Can you work these out from the model? Positions are in its coordinate system, mm. Face numbers are marked on the shaded views. A direction names the side the tool comes from. Round coordinates to 2 decimals unless told otherwise and drop trailing zeros. Order: outer loops, then holes, each group sorted by start corner. A loop starts at its lowest first (then second) coordinate and runs counter-clockwise, first axis right, second up. Notation, with made-up numbers: M -23.75,22 L 33.25,22 A25 cw 33.25,35 Z; hole C -2.5,6 d11. An arc over 180 degrees is marked long. One line per question, with ' | ' between items.
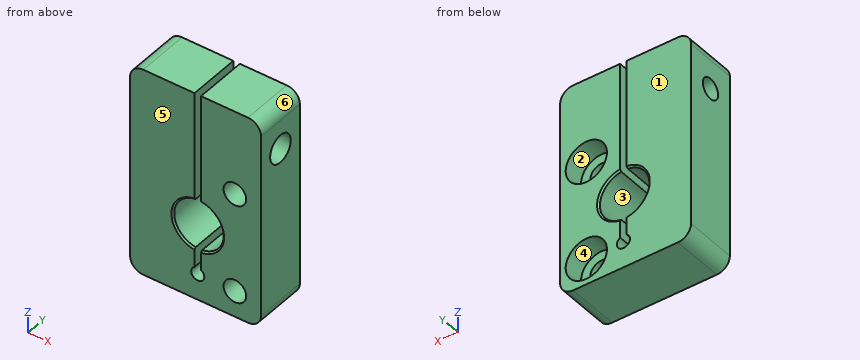
```python
from build123d import *

# Parameters (mm, degrees)
SKETCH1_W                            = 12.7
SKETCH1_H                            = 31.75
EXTRUDE1_DEPTH                       = 25.4
CBORE_FOR_M5_SHCS1_D                 = 5.5
CBORE_FOR_M5_SHCS1_DEPTH             = 12.7
CBORE_FOR_M5_SHCS1_CBORE_D           = 10
CBORE_FOR_M5_SHCS1_CBORE_DEPTH       = 5
CUT_EXTRUDE1_REACH                   = 14.7
F_17_64_0_26563_DIAMETER_HOLE1_D     = 6.747002
F_17_64_0_26563_DIAMETER_HOLE1_DEPTH = 14.55625
M6X1_0_TAPPED_HOLE1_D                = 5
M6X1_0_TAPPED_HOLE1_DEPTH            = 15.60625
FILLET1_R                            = 3.175
CHAMFER1_SIZE                        = 0.396875


with BuildPart() as part:
    # Sketch1 → Extrude1 (new body, symmetric)
    with BuildSketch(Plane(origin=(0, 0, 0), x_dir=(0, 1, 0), z_dir=(0, 0, 1))):
        Rectangle(SKETCH1_W, SKETCH1_H)
    extrude(amount=EXTRUDE1_DEPTH, both=True)

    # CBORE for M5 SHCS1
    with Locations(Plane(origin=(0, 6.35, 0), x_dir=(-1, 0, 0), z_dir=(0, 1, 0))):
        with Locations((-9.525, -19.05), (-9.525, 4.95)):
            CounterBoreHole(CBORE_FOR_M5_SHCS1_D / 2, CBORE_FOR_M5_SHCS1_CBORE_D / 2, CBORE_FOR_M5_SHCS1_CBORE_DEPTH, depth=CBORE_FOR_M5_SHCS1_DEPTH)

    # Sketch4 → Cut-Extrude1 (cut, up to next)
    with BuildSketch(Plane(origin=(0, 6.35, 0), x_dir=(1, 0, 0), z_dir=(0, 1, 0)), mode=Mode.PRIVATE) as cut_extrude1_sk1:
        with BuildLine():
            Line((-0.26875, 17.675184671), (-0.26875, 12.997264996))
            ThreePointArc((-0.26875, 12.997264996), (-5.475, 7.05), (-0.26875, 1.102735004))
            Line((-0.26875, 1.102735004), (-0.26875, -25.4))
            Line((-0.26875, -25.4), (1.31875, -25.4))
            Line((1.31875, -25.4), (1.31875, 1.102735004))
            ThreePointArc((1.31875, 1.102735004), (6.525, 7.05), (1.31875, 12.997264996))
            Line((1.31875, 12.997264996), (1.31875, 17.675184671))
            ThreePointArc((1.31875, 17.675184671), (0.525, 20.6375), (-0.26875, 17.675184671))
        make_face()
    cut_extrude1_tool1 = extrude(cut_extrude1_sk1.sketch, amount=-CUT_EXTRUDE1_REACH, mode=Mode.PRIVATE) & part.part
    add(cut_extrude1_tool1.solids().sort_by_distance((0.525, 6.35, -3.20917))[0], mode=Mode.SUBTRACT)

    # 17/64 (0.26563) Diameter Hole1
    with Locations(Plane(origin=(15.875, 0, 0), x_dir=(0, 0, -1), z_dir=(1, 0, 0))):
        with Locations((-15.175, 0)):
            Hole(F_17_64_0_26563_DIAMETER_HOLE1_D / 2, depth=F_17_64_0_26563_DIAMETER_HOLE1_DEPTH)

    # M6x1.0 Tapped Hole1
    with Locations(Plane(origin=(-0.26875, 0, 0), x_dir=(0, 0, -1), z_dir=(1, 0, 0))):
        with Locations((-15.175, 0)):
            Hole(M6X1_0_TAPPED_HOLE1_D / 2, depth=M6X1_0_TAPPED_HOLE1_DEPTH)

    # Fillet1
    fillet1_edges = [part.edges().sort_by_distance(p)[0] for p in [
        (15.875, 0, 25.4),
        (15.875, 0, -25.4),
        (-15.875, 0, -25.4),
        (-15.875, 0, 25.4),
    ]]
    fillet(fillet1_edges, radius=FILLET1_R)

    # Chamfer1
    chamfer1_edges = [part.edges().sort_by_distance(p)[0] for p in [
        (-5.475, 6.35, -7.05),
        (6.525, 6.35, -7.05),
        (6.525, -6.35, -7.05),
        (-5.475, -6.35, -7.05),
    ]]
    chamfer(chamfer1_edges, length=CHAMFER1_SIZE)


solid = part.part
```
(1) If we section it at A-A on y = 0: State how many separate pieces and enclosed holes the cut face has, plus the area to 3 significant figures.
Final values:
separate pieces: 3 | enclosed holes: 2 | area: 1,210 mm^2
(2) Please list where these lines run through material, in increasing order: probe 1 along Z at (x, y) = (8.5, -0.25); probe 2 along X at (y, z) = (1.5, -15) (3 decimals); probe 3 along Z at (x, y) = (8.5, 5.5). Write a range as [from, to].
Final values:
probe 1: [-25.4, -21.6], [-16.5, 2.4], [7.5, 11.81], [18.54, 25.4] | probe 2: [-15.875, -0.269], [1.319, 6.593], [12.457, 15.875] | probe 3: [-25.4, -23.94], [-14.16, 0.06], [9.84, 25.4]
(3) Will these pins go through, and if not, where does the flat tip stop? pin 1 Ø3 at (x, z) = (0.525, -19.05) entering from +Y; pin 2 Ø7 at (x, z) = (9.525, 4.95) entering from +Y.
Final values:
pin 1: through | pin 2: y = 1.35
(4) Thinking about a two-plate mould opening in X: for the marked faces 4, 5 and 6, which applies, released by +X, released by -X, zero draft, split by the parting line, or undercut?
Final values:
face 4: undercut | face 5: zero draft | face 6: released by +X
(5) If we section it at C-C on x = -11: Please give me the cut outline in (y, z) (3 decimals).
Final values:
outline: M -6.35,-25.4 L 6.35,-25.4 L 6.35,25.4 L -6.35,25.4 Z; hole C 0,15.175 d5
(6) On a 3-axis mill with a long thin cutter (end or side, diameter ignored), from which of +Z, -Z, +X, -X, +Y, -Y can I reach the whole of each face in a straight line? I mean the marked faces 1, 2 and 3. Say none if no direction works.
Final values:
face 1: +Z, -Z, +X, -X, +Y | face 2: +Y | face 3: +Y, -Y
